For this review, take the finished solid that the model builds, in its own axes (mm). A direction names the side the tool comes from. Give positions to 0.01 mm unless a question says otherwise; leave off trailing zeros. Write each loop counter-clockwise with the first axis right and the second up, starting at its lowest first coordinate (ties: lowest second). Pieces come first, ordered by that corner, then holes.
Q1. Mouldability with a two-part tool opening along Y and no side actions: class faces 1 (the flat face through (-1, 16, 0)), 2 (the cylindrical face through (35.49, -10.72, 1.57)), 3 (the flat face through (53, -27, 2)) as released by +Y, released by -Y, zero draft, split by the parting line, or undercut.
Q2. We need section A-A (x = 20.5). Write out the cut boundary in (y, z).
Q3. We need section D-D (y = -30). Write out the cut boundary in (x, z).
Q4. For line 1 (Y direction, x = -18, z = 2.4); line 2 (X direction, y = 1, z = 2.95); line 3 (Y direction, x = 27, z = 0.25), list the stretches that pass through material, from the lowest coordinate up.
Q5. We need section C-C (y = 11.5). Write out the cut boundary in (x, z).
Q6. Machinability: for faces 4 (the cylindrical face through (35.72, 10.49, 1.57)), 5 (the flat face through (-60, 0, 2)), which of the approach directions +Z, -Z, +X, -X, +Y, -Y give a long, thin tool a straight path to every point of the face, cutting with its end or side? Answer none if there is none.
```python
from build123d import *

# Parameters (mm, degrees)
SKETCH1_W           = 120
SKETCH1_H           = 70
SKETCH1_W_2         = 80
SKETCH1_H_2         = 30
BOSS_EXTRUDE1_DEPTH = 3.1
FILLET1_R           = 15
CHAMFER1_SIZE       = 15


with BuildPart() as part:
    # Sketch1 → Boss-Extrude1 (new body)
    with BuildSketch(Plane.XY):
        Rectangle(SKETCH1_W, SKETCH1_H)
        Rectangle(SKETCH1_W_2, SKETCH1_H_2, mode=Mode.SUBTRACT)
    extrude(amount=BOSS_EXTRUDE1_DEPTH)

    # Fillet1
    fillet1_edges = [part.edges().sort_by_distance(p)[0] for p in [
        (40, -15, 1.55),
        (40, 15, 1.55),
        (-40, 15, 1.55),
        (-40, -15, 1.55),
    ]]
    fillet(fillet1_edges, radius=FILLET1_R - 0.0001)  # a hair under: the kernel refuses the full size

    # Chamfer1
    chamfer1_edges = [part.edges().sort_by_distance(p)[0] for p in [
        (60, -35, 1.55),
        (60, 35, 1.55),
    ]]
    chamfer(chamfer1_edges, length=CHAMFER1_SIZE)


solid = part.part
```
Computed:
1. face 1: zero draft
1. face 2: undercut
1. face 3: released by -Y
2. outline: (-35, 0) - (-15, 0) - (-15, 3.1) - (-35, 3.1) - close; (15, 0) - (35, 0) - (35, 3.1) - (15, 3.1) - close
3. outline: (-60, 0) - (50, 0) - (50, 3.1) - (-60, 3.1) - close
4. line 1: y = -35 to -15, 15 to 35
4. line 2: x = -60 to -39.97, 39.97 to 60
4. line 3: y = -35 to -14.87, 14.87 to 35
5. outline: (-60, 0) - (-34.63, 0) - (-34.63, 3.1) - (-60, 3.1) - close; (34.63, 0) - (60, 0) - (60, 3.1) - (34.63, 3.1) - close
6. face 4: +Z, -Z
6. face 5: +Z, -Z, -X, +Y, -Y
